CAD build for the part. Positions are in the model's coordinates, mm. A direction names the side the tool comes from. Round coordinates to 2 decimals unless told otherwise and drop trailing zeros. Write each loop counter-clockwise with the first axis right and the second up, starting at its lowest first coordinate (ties: lowest second). Pieces come first, ordered by that corner, then holes. Notation, with made-up numbers: (-6, 2.25) - (51, 2.25) arc R25 ccw to (51, 16.25) - close; hole circle Ø5 at (39.25, -39). An arc over 180 degrees is marked (long way). Put each result on its own line as item: value. Start each with the question number.
Item 1: Pin check, flat tips, straight feed: pin 1 Ø1.5 at (x, z) = (32.5, 33.5) entering from +Y; pin 2 Ø6 at (x, z) = (-9.779, 0) entering from +Y (3 decimals); pin 3 Ø1.5 at (x, y) = (8.5, 2) entering from -Z. Stop position of each tip, or through.
Item 2: Drill centre lines: line 1 (X direction, y = 0.95, z = 0); line 2 (Z direction, x = 0, y = 2.2); line 3 (X direction, y = 1.5, z = -0.5). Where is each one in solid material? Low to high. Write a range as from..to.
Item 3: 3-axis set-ups, long thin cutter, end or side, ignore diameter. For faces 4 (the flat face through (9, 3.175, 9)), 5 (the cylindrical face through (29.082, 1.565, -29.192)): which of +Z, -Z, +X, -X, +Y, -Y reach the whole face in a straight line?
Item 4: Mould opens along Z. For faces 1 (the flat face through (9, 0, 9)), 2 (the cylindrical face through (20.364, 1.565, -31.37)), 3 (the cylindrical face through (42.397, 1.61, -13.352)) say: released by +Z, released by -Z, zero draft, split by the parting line, or undercut.
Item 5: Cut at D-D (z = 36.83). Give the cut face in (x, y) (3 decimals), and give its area (3 significant figures).
Item 6: Cut at B-B (z = 0). Give the cut face in (x, y) (3 decimals), and give its area (3 significant figures).
Item 7: Cut at C-C (y = 2.4). Count the separate pieces of the cut face and the enclosed holes in it, and give its area (3 significant figures).
Item 8: Cut at A-A (x = 0). Give the cut face in (y, z) (3 decimals).
Autodesk Inventor part; units mm, degrees
ref_plane "YZ Plane" through (0, 0, 0) normal (1, 0, 0) x (0, 1, 0)
ref_plane "XZ Plane" through (0, 0, 0) normal (0, 1, 0) x (-1, 0, 0)
ref_plane "XY Plane" through (0, 0, 0) normal (0, 0, 1) x (1, 0, 0)
ref_plane "Work Plane1" through (0, 1.5875, 0) normal (0, 1, 0) x (1, 0, 0)
sketch "Sketch1" plane through (0, 1.5875, 0) normal (0, 1, 0) x (1, 0, 0)
  circle A0 centre (0, 0) radius 44.45
  circle A1 centre (0, -9.779) radius 1.778 construction
  circle A2 centre (-9.779, 0) radius 1.778 construction
  circle A3 centre (0, 9.779) radius 1.778 construction
  circle A4 centre (9.779, 0) radius 1.778 construction
  circle A5 centre (0, 0) radius 6.35 construction
  circle A6 centre (0, -9.779) radius 1.9304
  circle A7 centre (-9.779, 0) radius 1.9304
  circle A8 centre (0, 9.779) radius 1.9304
  circle A9 centre (9.779, 0) radius 1.9304
  circle A10 centre (0, 0) radius 6.477
  circle A11 centre (0, 0) radius 34.925 construction
  circle A12 centre (0, -36.83) radius 1.9304
  circle A13 centre (0, 36.83) radius 1.9304
  line L0 (0, 0) -> (31.4309, 31.4309) construction
  line L1 (0, 0) -> (44.45, 0) construction
  line L2 (28.8087, 22.5367) -> (28.1119, 23.6217)
  line L3 (22.1752, 26.6653) -> (23.6324, 28.1226)
  line L4 (23.6324, 28.1226) -> (22.5367, 28.8087)
  line L5 (21.5127, 27.0801) -> (22.1752, 26.6653)
  line L6 (28.1119, 23.6217) -> (26.6653, 22.1752)
  arc A14 (28.8087, 22.5367) -> (30.8149, 23.7252) centre (29.8118, 23.131) ccw
  arc A15 (23.7252, 30.8149) -> (22.5367, 28.8087) centre (23.131, 29.8118) ccw
  arc A16 (24.7492, 32.5435) -> (21.5127, 27.0801) centre (23.131, 29.8118) ccw
  arc A17 (27.0801, 21.5127) -> (32.5435, 24.7492) centre (29.8118, 23.131) ccw
  arc A18 (30.8149, 23.7252) -> (23.7252, 30.8149) centre (13.4217, 13.4217) ccw
  arc A19 (32.5435, 24.7492) -> (24.7492, 32.5435) centre (13.4217, 13.4217) ccw
  line L7 (27.0801, 21.5127) -> (26.6653, 22.1752)
  point P0 (24.7492, 32.5435)
  dimension "d1" = 88.9
  dimension "d2" = 3.8608
  dimension "d3" = 3.8608
  dimension "d5" = 3.8608
  dimension "d6" = 12.954
  dimension "d7" = 69.85
  dimension "d8" = 3.8608
  dimension "d10" = 3.8608
  dimension "d11" = 36.83
  dimension "d12" = 45
  dimension "d13" = 36.83
extrude "Extrusion1" add sketch "Sketch1" along normal mid plane 3.175
properties part number "3_5 in spool outer plate"
Output values:
1. pin 1: through
1. pin 2: y = 3.175
1. pin 3: z = -43.77
2. line 1: -44.45..-11.71, -7.85..-6.48, 6.48..7.85, 11.71..44.45
2. line 2: -44.45..-38.76, -34.9..-11.71, -7.85..-6.48, 6.48..7.85, 11.71..34.9, 38.76..44.45
2. line 3: -44.45..-11.64, -7.91..-6.46, 6.46..7.91, 11.64..44.45
3. face 4: +Z, -Z, +X, -X, +Y
3. face 5: +Y, -Y
4. face 1: zero draft
4. face 2: undercut
4. face 3: split by the parting line
5. outline: (-24.887, 0) - (-1.93, 0) - (-1.93, 3.175) - (-24.887, 3.175) - close; (1.93, 0) - (24.887, 0) - (24.887, 3.175) - (1.93, 3.175) - close
5. area: 146 mm2
6. outline: (-44.45, 0) - (-11.709, 0) - (-11.709, 3.175) - (-44.45, 3.175) - close; (-7.849, 0) - (-6.477, 0) - (-6.477, 3.175) - (-7.849, 3.175) - close; (6.477, 0) - (7.849, 0) - (7.849, 3.175) - (6.477, 3.175) - close; (11.709, 0) - (44.45, 0) - (44.45, 3.175) - (11.709, 3.175) - close
6. area: 217 mm2
7. separate pieces: 1
7. enclosed holes: 8
7. area: 5,950 mm2
8. outline: (0, -44.45) - (3.175, -44.45) - (3.175, -38.76) - (0, -38.76) - close; (0, -34.9) - (3.175, -34.9) - (3.175, -11.709) - (0, -11.709) - close; (0, -7.849) - (3.175, -7.849) - (3.175, -6.477) - (0, -6.477) - close; (0, 6.477) - (3.175, 6.477) - (3.175, 7.849) - (0, 7.849) - close; (0, 11.709) - (3.175, 11.709) - (3.175, 34.9) - (0, 34.9) - close; (0, 38.76) - (3.175, 38.76) - (3.175, 44.45) - (0, 44.45) - close
